Can you work these out from the model? Positions are in its coordinate system, mm. A direction names the side the tool comes from. Give positions to 0.01 mm unless a question says otherwise; leave off trailing zeros. Order: outer loops, then holes, each group sorted by start corner. A loop starts at its lowest first (then second) coordinate and runs counter-clockwise, first axis right, second up. Notation, with made-up numbers: M -22,37.25 L -6,37.25 A22 ccw -6,56.25 Z; hole C 39,34.25 d4. An arc over 180 degrees is marked long. Write each question's results on one line, items separated by ' | '.
from build123d import *

# Parameters (mm, degrees)
EXTRUDE_1_DEPTH     = 3
CUT_EXTRUDE_4_DEPTH = 4
SKETCH_12_R         = 15
SKETCH_12_R_2       = 5.9
EXTRUDE_2_DEPTH     = 2.6
SKETCH_13_R         = 15
SKETCH_13_R_2       = 6.75
EXTRUDE_3_DEPTH     = 1.1
SKETCH_14_R         = 1.2
CUT_EXTRUDE_5_DEPTH = 7.7
FILLET_1_R          = 1


with BuildPart() as part:
    # 스케치1 → 보스-돌출1 (new body)
    with BuildSketch(Plane.XY):
        with BuildLine():
            Line((-5, -6.9), (-6.9, -6.9))
            Line((-6.9, -6.9), (-6.9, 6.9))
            Line((-6.9, 6.9), (6.9, 6.9))
            Line((6.9, 6.9), (6.9, -6.9))
            Line((6.9, -6.9), (5, -6.9))
            Line((5, -6.9), (5, -14.142135624))
            ThreePointArc((5, -14.142135624), (0, 15), (-5, -14.142135624))
            Line((-5, -14.142135624), (-5, -6.9))
        make_face()
    extrude(amount=EXTRUDE_1_DEPTH)

    # 스케치11 → 컷-돌출4 (cut, through all)
    with BuildSketch(Plane.XY.offset(3)):
        with BuildLine():
            Line((5.8, -1.8), (-5.8, -1.8))
            ThreePointArc((-5.8, -1.8), (-7.6, 0), (-5.8, 1.8))
            Line((-5.8, 1.8), (5.8, 1.8))
            ThreePointArc((5.8, 1.8), (7.6, 0), (5.8, -1.8))
        make_face()
    extrude(amount=-CUT_EXTRUDE_4_DEPTH, mode=Mode.SUBTRACT)

    # 스케치12 → 보스-돌출2 (add)
    with BuildSketch(Plane.XY.offset(3)):
        Circle(SKETCH_12_R)
        Circle(SKETCH_12_R_2, mode=Mode.SUBTRACT)
    extrude(amount=EXTRUDE_2_DEPTH)

    # 스케치13 → 보스-돌출3 (add)
    with BuildSketch(Plane.XY.offset(5.6)):
        Circle(SKETCH_13_R)
        Circle(SKETCH_13_R_2, mode=Mode.SUBTRACT)
    extrude(amount=EXTRUDE_3_DEPTH)

    # 스케치14 → 컷-돌출5 (cut, through all)
    with BuildSketch(Plane.XY.offset(6.7)):
        with Locations((10.825317547, 6.25)):
            Circle(SKETCH_14_R)
        with Locations((-10.825317547, 6.25)):
            Circle(SKETCH_14_R)
        with Locations((10.825317547, -6.25)):
            Circle(SKETCH_14_R)
        with Locations((-10.825317547, -6.25)):
            Circle(SKETCH_14_R)
    extrude(amount=-CUT_EXTRUDE_5_DEPTH, mode=Mode.SUBTRACT)

    # 필렛1
    fillet_1_edges = [part.edges().sort_by_distance(p)[0] for p in [
        (-5, -6.9, 1.5),
        (5, -6.9, 1.5),
    ]]
    fillet(fillet_1_edges, radius=FILLET_1_R)


solid = part.part
(1) Imagine slicing it at B-B, the plane z = 1.75. Write out the boundary of the cut face in (x, y).
Data:
outline: M -6.9,-6.9 L -6.9,-1.42 A1.8 cw -6.9,1.42 L -6.9,6.9 L 6.9,6.9 L 6.9,1.42 A1.8 cw 6.9,-1.42 L 6.9,-6.9 L 6,-6.9 A1 ccw 5,-7.9 L 5,-14.14 A15 ccw long -5,-14.14 L -5,-7.9 A1 ccw -6,-6.9 Z; hole C -10.83,-6.25 d2.4; hole C -10.83,6.25 d2.4; hole C 10.83,-6.25 d2.4; hole C 10.83,6.25 d2.4
(2) Imagine slicing it at A-A, the plane x = 0. Write out the boundary of the cut face in (y, z).
Data:
outline: M -15,3 L -5.9,3 L -5.9,5.6 L -6.75,5.6 L -6.75,6.7 L -15,6.7 Z; M 5.9,3 L 6.9,3 L 6.9,0 L 15,0 L 15,6.7 L 6.75,6.7 L 6.75,5.6 L 5.9,5.6 Z
(3) We'd pull the mould along X, two halves only. Please class faces 1 (the face through (-0.2, 7.1, 0)), 2 (the face through (6.9, -4, 1)), 3 (the face through (3.5, -5, 5.6)): +X half, -X half, draft (parallel to the pull), parting line (faces both ways), or undercut.
Data:
face 1: draft | face 2: undercut | face 3: undercut
(4) Will these pins go through, and if not, where does the flat tip stop? P1, Ø4, axis at x = 10.5, z = 5.5, coming from the +Y side; P2, Ø3, axis at x = 10.83, y = -6.25, coming from the +Z side; P3, Ø1.5, axis at y = -3.5, z = 2, coming from the +X side; P4, Ø0.9, axis at y = 5, z = 1, coming from the -X side.
Data:
P1: stops at y = 12.36 | P2: stops at z = 6.7 | P3: stops at x = 14.75 | P4: stops at x = -14.29
(5) Imagine slicing it at D-D, the plane y = 5.5. Write out the boundary of the cut face in (x, z).
Data:
outline: M -13.96,0 L -11.76,0 L -11.76,6.7 L -13.96,6.7 Z; M -9.89,0 L -6.9,0 L -6.9,3 L -2.14,3 L -2.14,5.6 L -3.91,5.6 L -3.91,6.7 L -9.89,6.7 Z; M 2.14,3 L 6.9,3 L 6.9,0 L 9.89,0 L 9.89,6.7 L 3.91,6.7 L 3.91,5.6 L 2.14,5.6 Z; M 11.76,0 L 13.96,0 L 13.96,6.7 L 11.76,6.7 Z
(6) For faces 4 (the face through (-1.46, -6.59, 6.14)), 5 (the face through (5, -11, 1)), 6 (the face through (-5.285, -7.201, 1.521)), which set-ups out of +Z, -Z, +X, -X, +Y, -Y let a thin tool reach every point of the face, with its end or its side?
Data:
face 4: +Z | face 5: -Z, -Y | face 6: -Z
(7) I need wall thicknesses on L1, parallel to Y at x = 0, z = 6.4; L2, parallel to X at y = 6.5, z = 2.75; L3, parallel to Z at x = 3.5, y = -6.5. Which ranges of each line are inside material? Lowest first, please. Write a range as from..to.
Data:
L1: y = -15..-6.75, 6.75..15 | L2: x = -13.52..-12, -9.65..-6.9, 6.9..9.65, 12..13.52 | L3: z = 3..6.7
(8) Imagine slicing it at C-C, the plane z = 4. Write out the boundary of the cut face in (x, y).
Data:
outline: C 0,0 d30; hole C -10.83,-6.25 d2.4; hole C -10.83,6.25 d2.4; hole C 0,0 d11.8; hole C 10.83,-6.25 d2.4; hole C 10.83,6.25 d2.4
